from build123d import *

# Parameters (mm, degrees)
BOSS_EXTRUDE1_DEPTH          = 44.45
BOSS_EXTRUDE1_DEPTH_BACK     = 9.525
SKETCH1_W                    = 51.1175
SKETCH1_H                    = 33.3502
SKETCH2_W                    = 51.1175
SKETCH2_H                    = 20.6502
CUT_EXTRUDE1_DEPTH           = 36.195
CUT_EXTRUDE2_DEPTH           = 62.166069365
CUT_EXTRUDE2_DEPTH_BACK      = 62.166069365
FILLET3_R                    = 6.35
F_3_8_0_375_DIAMETER_HOLE1_D = 9.525
F_3_8_0_375_DIAMETER_HOLE2_D = 9.525


with BuildPart() as part:
    # Sketch1 → Boss-Extrude1 (new, two sides: drawn at the far end of the back side and taken through both)
    with BuildSketch(Plane(origin=(0, 0, 0), x_dir=(1, 0, 0), z_dir=(0, 1, 0)).offset(-BOSS_EXTRUDE1_DEPTH_BACK)):
        Rectangle(SKETCH1_W, SKETCH1_H)
    extrude(amount=BOSS_EXTRUDE1_DEPTH + BOSS_EXTRUDE1_DEPTH_BACK)

    # Sketch2 → Cut-Extrude1 (cut)
    with BuildSketch(Plane(origin=(0, 44.45, 0), x_dir=(1, 0, 0), z_dir=(0, 1, 0))):
        Rectangle(SKETCH2_W, SKETCH2_H)
    extrude(amount=-CUT_EXTRUDE1_DEPTH, mode=Mode.SUBTRACT)

    # Sketch3 → Cut-Extrude2 (cut, two sides: drawn at the far end of the back side and taken through both)
    with BuildSketch(Plane(origin=(0, 0, -16.6751), x_dir=(-1, 0, 0), z_dir=(0, 0, -1)).offset(-CUT_EXTRUDE2_DEPTH_BACK)):
        Polygon((25.55875, 44.45), (9.525, 44.45), (25.55875, 9.525), align=None)
        Polygon((-25.55875, 9.525), (-9.525, 44.45), (-25.55875, 44.45), align=None)
    extrude(amount=CUT_EXTRUDE2_DEPTH + CUT_EXTRUDE2_DEPTH_BACK, mode=Mode.SUBTRACT)

    # Fillet3
    fillet3_edges = [part.edges().sort_by_distance(p)[0] for p in [
        (-9.525, 44.45, -13.5001),
        (-9.525, 44.45, 13.5001),
        (9.525, 44.45, -13.5001),
        (9.525, 44.45, 13.5001),
    ]]
    fillet(fillet3_edges, radius=FILLET3_R)

    # 3/8 (0.375) Diameter Hole1 (through all)
    with Locations(Plane.XY.offset(16.6751)):
        with Locations((0, 25.161662577)):
            Hole(F_3_8_0_375_DIAMETER_HOLE1_D / 2)

    # 3/8 (0.375) Diameter Hole2 (through all)
    with Locations(Plane.ZY.offset(25.55875)):
        with Locations((-8.5, 0), (8.5, 0)):
            Hole(F_3_8_0_375_DIAMETER_HOLE2_D / 2)


solid = part.part
Read the model definition and answer for the solid it produces. Units are mm, in the model's axes. A direction names the side the tool comes from. Coordinates: 2 decimals unless noted, no trailing zeros. Loops run counter-clockwise (first coordinate to the right, second up) from the corner with the lowest first, then second, coordinate; pieces in that order, holes last. Notation, with made-up numbers: (-27.75, 70.25) - (-3.75, 70.25) arc R9 ccw to (-3.75, 79.25) - close; hole circle Ø7 at (35, 66.25). An arc over 180 degrees is marked (long way). Answer in a Markdown table with one row per item.
Q1. Find section A-A on z = 8.5. Write down the section's boundary in (x, y) (1 decimal), plus the area to 3 significant figures.
Here are the results:
| item | result |
|---|---|
| outline | (-25.6, -9.5) - (25.6, -9.5) - (25.6, -4.8) - (-25.6, -4.8) - close; (-25.6, 4.8) - (25.6, 4.8) - (25.6, 8.3) - (-25.6, 8.3) - close |
| area | 422 mm^2 |
Q2. Straight lines are drawn through the part: line 1 along Z through (x, y) = (-8, 23); line 2 along Y through (x, z) = (0, 14) (3 decimals); line 3 along Z through (x, y) = (3.5, 1). For each, find the intervals that lie inside material, in ascending order. Write a range as [from, to].
Here are the results:
| item | result |
|---|---|
| line 1 | z = [-16.68, -10.33], [10.33, 16.68] |
| line 2 | y = [-9.525, 20.399], [29.924, 44.45] |
| line 3 | z = [-16.68, -13.16], [-3.84, 3.84], [13.16, 16.68] |
Q3. The mould has two halves that part along Z. Classify faces 1 (the flat face through (-18.29, 25.36, -13.46)), 2 (the flat face through (0, 19, 10.325)), 3 (the flat face through (0, 11, 16.675)): pulls with the +Z half, pulls with the -Z half, needs draft (parallel to the pull), parting line crosses it, or undercut.
Here are the results:
| item | result |
|---|---|
| face 1 | needs draft |
| face 2 | undercut |
| face 3 | pulls with the +Z half |
Q4. Find section D-D on y = 14.5. Write down the section's boundary in (x, z).
Here are the results:
| item | result |
|---|---|
| outline | (-23.27, -16.68) - (23.27, -16.68) - (23.27, -10.33) - (-23.27, -10.33) - close; (-23.27, 10.33) - (23.27, 10.33) - (23.27, 16.68) - (-23.27, 16.68) - close |
Q5. Find section C-C on y = 0. Write down the section's boundary in (x, z).
Here are the results:
| item | result |
|---|---|
| outline | (-25.56, -16.68) - (25.56, -16.68) - (25.56, -13.26) - (-25.56, -13.26) - close; (-25.56, -3.74) - (25.56, -3.74) - (25.56, 3.74) - (-25.56, 3.74) - close; (-25.56, 13.26) - (25.56, 13.26) - (25.56, 16.68) - (-25.56, 16.68) - close |
Q6. For faces 4 (the flat face through (0, 8.255, 0)), 5 (the cylindrical face through (-8.92, 43.42, -13.54)), determine the directions among +Z, -Z, +X, -X, +Y, -Y from which every point of the face is accessible in a straight line to the end or side of a thin tool.
Here are the results:
| item | result |
|---|---|
| face 4 | +X, -X, +Y |
| face 5 | +Z, -Z, -X, +Y |
Q7. Given P1, Ø6, axis at y = 24, z = -13, coming from the +X side; P2, Ø5, axis at x = -12.5, z = 6.5, coming from the +Y side (3 decimals); P3, Ø15, axis at x = 0, y = 25.16, coming from the -Z side, each flat-ended and moving along its own axis, determine where each tip first touches the part or whether it passes through.
Here are the results:
| item | result |
|---|---|
| P1 | stops at x = 20.29 |
| P2 | stops at y = 8.255 |
| P3 | stops at z = -16.68 |
Q8. Find section B-B on x = 0. Count the separate pieces of the cut face and the enclosed holes in it, plus the area to 3 significant figures.
Here are the results:
| item | result |
|---|---|
| separate pieces | 3 |
| enclosed holes | 2 |
| area | 789 mm^2 |
